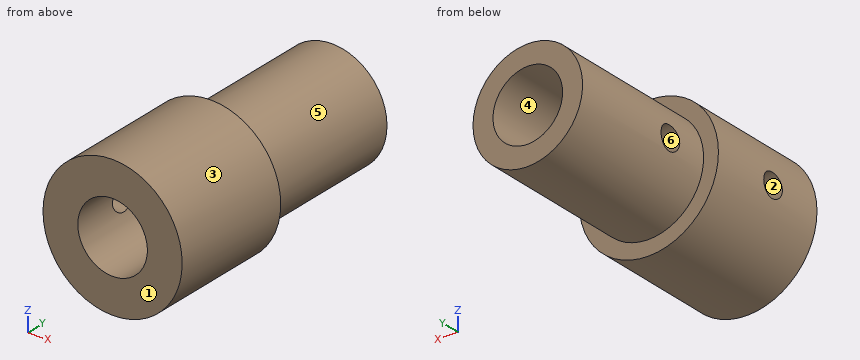
Autodesk Inventor part; units mm, degrees
ref_plane "YZ Plane" through (0, 0, 0) normal (1, 0, 0) x (0, 1, 0)
ref_plane "XZ Plane" through (0, 0, 0) normal (0, 1, 0) x (-1, 0, 0)
ref_plane "XY Plane" through (0, 0, 0) normal (0, 0, 1) x (1, 0, 0)
sketch "Sketch1" plane through (0, 0, 0) normal (0, 1, 0) x (-1, 0, 0)
  circle A0 centre (0, 0) radius 6.35
  circle A1 centre (0, 0) radius 3.175
  dimension "d0" = 12.7
  dimension "d1" = 6.35
extrude "Extrusion1" add sketch "Sketch1" along normal blind 25.4
sketch "Sketch2" plane through (0, 25.4, 0) normal (0, 1, 0) x (1, 0, 0)
  circle A0 centre (0, 0) radius 6.35
  circle A1 centre (0, 0) radius 5
  dimension "d4" = 10
extrude "Extrusion2" cut sketch "Sketch2" against normal blind 14
sketch "Sketch3" plane through (0, 0, 0) normal (1, 0, 0) x (0, 1, 0)
  point P0 (0, 0)
  point P1 (5.08, 0)
  point P2 (15.24, 0)
  dimension "d7" = 5.08
  dimension "d8" = 15.24
hole "Hole1" at (0, 5.08, 0) at (0, 15.24, 0) direction (-1, 0, 0) diameter 2.159 end through all
properties part number "motorCoupling"
For this review, take the finished solid that the model builds, in its own axes (mm). Face numbers are marked on the shaded views. A direction names the side the tool comes from. Give positions to 0.01 mm unless a question says otherwise; leave off trailing zeros. Loops run counter-clockwise (first coordinate to the right, second up) from the corner with the lowest first, then second, coordinate; pieces in that order, holes last. Notation, with made-up numbers: M 42.5,-39.5 L 78.5,-39.5 A21 ccw 78.5,-34.5 Z; hole C 30.25,32.5 d4. An arc over 180 degrees is marked long. One line per item, written item: value. Start each with the question number.
Q1. For L1, parallel to Z at x = 0, y = 16 (3 decimals); L2, parallel to X at y = 12.75, z = 1.75; L3, parallel to Z at x = 0, y = 5.5 (3 decimals), list the stretches that pass through material, from the lowest coordinate up.
Q2. Clearance check with flat-ended pins moving along their axes: pin 1 Ø1.5 at (x, y) = (2.5, 3) entering from +Z; pin 2 Ø1.5 at (x, y) = (4, 9.5) entering from -Z; pin 3 Ø4 at (x, z) = (-4.5, 3.5) entering from +Y; pin 4 Ø2 at (x, y) = (4.5, 13) entering from +Z. State where each tip first meets the part, or that it passes through.
Q3. Add section B-B (x = 0). Give the boundary of the cut face in (y, z) (3 decimals).
Q4. Add section A-A (z = 0). Count the separate pieces of the cut face and the enclosed holes in it, and give its area (3 significant figures).
Q5. Draft analysis for pull direction Z (two halves, no side actions). For the marked faces 1, 2 and 3, state which applies: released by +Z, released by -Z, zero draft, split by the parting line, or undercut.
Q6. Add section C-C (y = 7.5). Give the boundary of the cut face in (x, z) (3 decimals), and give its area (3 significant figures).
Q7. Add section D-D (x = -3.5). Give the boundary of the cut face in (y, z), and give its area (3 significant figures).
Q8. Machinability: for the marked faces 4, 5 and 6, which of the approach directions +Z, -Z, +X, -X, +Y, -Y give a long, thin tool a straight path to every point of the face, cutting with its end or side? Answer none if there is none.
Reply:
1. L1: -5 to -3.175, 3.175 to 5
1. L2: -4.68 to -2.65, 2.65 to 4.68
1. L3: -6.35 to -3.175, 3.175 to 6.35
2. pin 1: z = 6.1
2. pin 2: z = -5.46
2. pin 3: y = 25.4
2. pin 4: z = 3.57
3. outline: M 0,-6.35 L 11.4,-6.35 L 11.4,-5 L 25.4,-5 L 25.4,-3.175 L 0,-3.175 Z; M 0,3.175 L 25.4,3.175 L 25.4,5 L 11.4,5 L 11.4,6.35 L 0,6.35 Z
4. separate pieces: 4
4. enclosed holes: 0
4. area: 113 mm²
5. face 1: zero draft
5. face 2: undercut
5. face 3: split by the parting line
6. outline: C 0,0 d12.7; hole C 0,0 d6.35
6. area: 95.0 mm²
7. outline: M 0,-5.3 L 11.4,-5.3 L 11.4,-3.57 L 25.4,-3.57 L 25.4,3.57 L 11.4,3.57 L 11.4,5.3 L 0,5.3 Z; hole C 5.08,0 d2.16; hole C 15.24,0 d2.16
7. area: 213 mm²
8. face 4: +Y, -Y
8. face 5: +Y
8. face 6: -X
